from build123d import *

# Parameters (mm, degrees)
F0_W     = 374
F0_H     = 212
F1_DEPTH = 10
F2_W     = 338
F2_H     = 176
F3_DEPTH = 187
F4_W     = 135.732657
F4_H     = 50
F5_DEPTH = 50
F7_D     = 6
F7_DEPTH = 10
F8_D     = 6.5
F8_DEPTH = 10


with BuildPart() as f1:
    # F0 (on Top) → F1 (new body)
    with BuildSketch(Plane.XY):
        Rectangle(F0_W, F0_H)
    extrude(amount=F1_DEPTH)

    # F2 (on face) → F3 (join)
    with BuildSketch(Plane(origin=(0, 0, 0), x_dir=(1, 0, 0), z_dir=(0, 0, -1))):
        Rectangle(F2_W, F2_H)
    extrude(amount=F3_DEPTH)

    # F4 (on face) → F5 (cut)
    with BuildSketch(Plane.XY.offset(10)):
        with Locations((10.02105, -38.9)):
            Rectangle(F4_W, F4_H)
    extrude(amount=-F5_DEPTH, mode=Mode.SUBTRACT)

    # F7
    with Locations(Plane.XY.offset(10)):
        with Locations((-167, 96), (-167, -96), (167, -96), (167, 96), (-10, 96), (10, -96)):
            Hole(F7_D / 2, depth=F7_DEPTH)

    # F8
    with Locations(Plane.XY.offset(10)):
        with Locations((-177, 96), (-177, -96), (0, -96), (0, 96), (177, 96), (177, -96)):
            Hole(F8_D / 2, depth=F8_DEPTH)


solid = f1.part
The listing builds one solid part. Answer for the finished solid, in the listing's coordinates (mm). A direction names the side the tool comes from. Give positions to 0.01 mm unless a question says otherwise; leave off trailing zeros. Write each loop counter-clockwise with the first axis right and the second up, starting at its lowest first coordinate (ties: lowest second). Pieces come first, ordered by that corner, then holes. Notation, with made-up numbers: (-9.75, 38.5) - (-1.75, 38.5) arc R20 ccw to (-1.75, 52.5) - close; hole circle Ø5 at (20, -4.5). An arc over 180 degrees is marked (long way). Use a Markdown table: item, result.
1. Section D-D on z = -88.5 is taken. Write down the section's boundary in (x, y), plus the area to 3 significant figures.
Values follow:
| item | result |
|---|---|
| outline | (-169, -88) - (169, -88) - (169, 88) - (-169, 88) - close |
| area | 59,500 mm² |
2. Find the intervals of material crossed by probe 1 along Y at (x, z) = (177, 2.5); probe 2 along X at (y, z) = (-27, -16.5); probe 3 along Y at (x, z) = (76.5, -8), in increasing order. Write a range as from..to.
Values follow:
| item | result |
|---|---|
| probe 1 | y = -106..-99.25, -92.75..92.75, 99.25..106 |
| probe 2 | x = -169..-57.85, 77.89..169 |
| probe 3 | y = -88..-63.9, -13.9..88 |
3. Section B-B on y = 42 is taken. Write down the section's boundary in (x, z), plus the area to 3 significant figures.
Values follow:
| item | result |
|---|---|
| outline | (-187, 0) - (-169, 0) - (-169, -187) - (169, -187) - (169, 0) - (187, 0) - (187, 10) - (-187, 10) - close |
| area | 66,900 mm² |
4. Section A-A on z = -9.5 is taken. Write down the section's boundary in (x, y).
Values follow:
| item | result |
|---|---|
| outline | (-169, -88) - (169, -88) - (169, 88) - (-169, 88) - close; hole (-57.85, -63.9) - (77.89, -63.9) - (77.89, -13.9) - (-57.85, -13.9) - close |
5. Each of these flat-tipped pins is pushed along its axis until it touches: P1, Ø2, axis at x = -100, z = -43, coming from the +Y side; P2, Ø8, axis at x = -167, y = 96, coming from the -Z side; P3, Ø6, axis at x = 0, y = 96, coming from the +Z side; P4, Ø4, axis at x = -28, z = -136, coming from the -Y side. Where does it stop, or does it pass through?
Values follow:
| item | result |
|---|---|
| P1 | stops at y = 88 |
| P2 | stops at z = 0 |
| P3 | passes through |
| P4 | stops at y = -88 |
6. A tool of negligible diameter and unlimited length cuts with its end or side. For faces 1 (the flat face through (187, -1, 5)), 2 (the flat face through (-3, 106, 5)), 3 (the flat face through (9, -63.9, -15)), 4 (the flat face through (169, 1, -92)), 5 (the flat face through (-2, -88, -92)), from which of +Z, -Z, +X, -X, +Y, -Y can it reach the whole face along a straight path? Write none if from no direction.
Values follow:
| item | result |
|---|---|
| face 1 | +Z, -Z, +X, +Y, -Y |
| face 2 | +Z, -Z, +X, -X, +Y |
| face 3 | +Z |
| face 4 | -Z, +X, +Y, -Y |
| face 5 | -Z, +X, -X, -Y |
7. For a pull along Y with two mould halves and no side action, classify faces 6 (the flat face through (9, -13.9, -15)), 7 (the flat face through (-169, 1, -92)), 8 (the flat face through (-2, 88, -92)) as released by +Y, released by -Y, zero draft, split by the parting line, or undercut.
Values follow:
| item | result |
|---|---|
| face 6 | undercut |
| face 7 | zero draft |
| face 8 | released by +Y |
8. Section C-C on x = -111.5 is taken. Write down the section's boundary in (y, z).
Values follow:
| item | result |
|---|---|
| outline | (-106, 0) - (-88, 0) - (-88, -187) - (88, -187) - (88, 0) - (106, 0) - (106, 10) - (-106, 10) - close |
